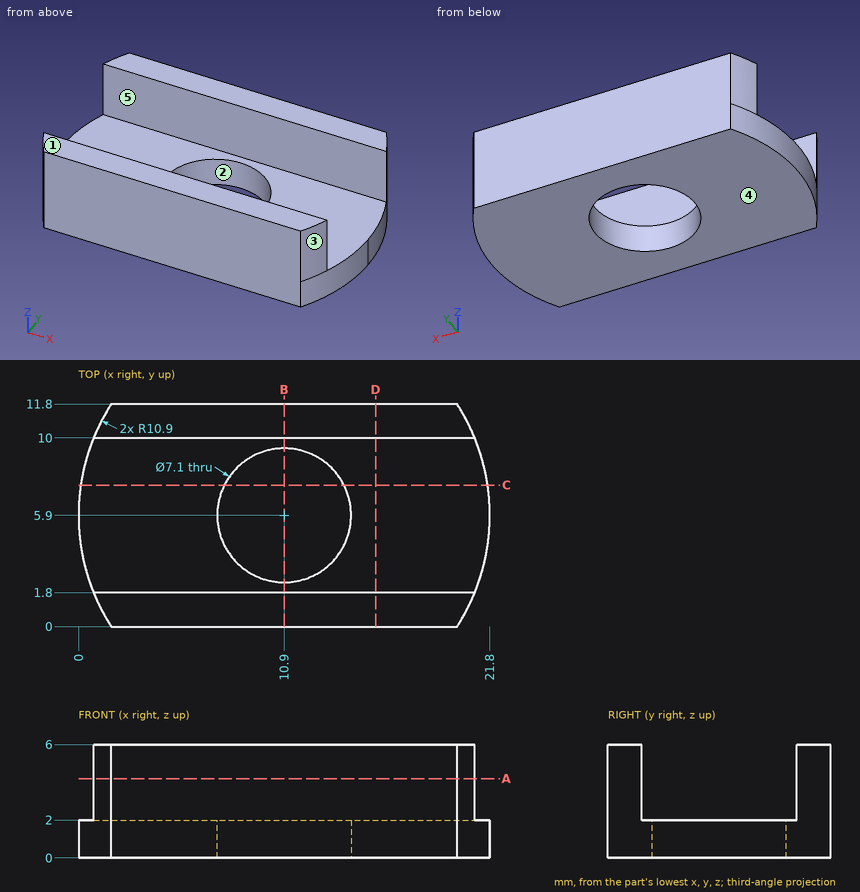
Source: three-view drawing plus pictorial views. Frame: mm from the lowest corner of the part. A direction names the side the tool comes from. Coordinates: 2 decimals unless noted, no trailing zeros. Order: outer loops, then holes, each group sorted by start corner. A loop starts at its lowest first (then second) coordinate and runs counter-clockwise, first axis right, second up. Notation, with made-up numbers: M 54.5,-3.75 L 104.5,-3.75 A15 ccw 104.5,25.25 Z; hole C 56.5,23.5 d9. An arc over 180 degrees is marked long. Write each question's results on one line, items separated by ' | '. Start each with the question number.
1. Section C-C, the plane y = 7.5. Return the cut outline in (x, z).
2. Section A-A, the plane z = 4.2. Return the cut outline in (x, y) (1 decimal), then the cut area to 3 significant figures.
3. Pin query (flat end, axial travel): pin 1 (1 mm diameter, centred on y = 10.5, z = 2, fed in from -X); pin 2 (5 mm diameter, centred on x = 3, y = 7.5, fed in from -Z); pin 3 (1.5 mm diameter, centred on y = 10.5, z = 1, fed in from -X). Return the tip coordinate at first contact, or that it passes through.
4. Reachability of the marked faces 4 and 5 from +Z, -Z, +X, -X, +Y, -Y: full face, straight path, thin tool, end or side. Return the list, or none.
5. Section D-D, the plane x = 15.75. Return the cut outline in (y, z).
6. Section B-B, the plane x = 10.9. Return the cut outline in (y, z), then the cut area to 3 significant figures.
7. Draft query along X for the marked faces 1, 2 and 3. Return one class per face: +X half, -X half, draft (parallel to the pull), parting line (faces both ways), or undercut.
8. Material intervals for L1, parallel to Y at x = 4.75, z = 2.35; L2, parallel to Y at x = 10.9, z = 1.25; L3, parallel to Z at x = 17.25, y = 3.5, sorted ascending.
Solution:
1) outline: M 0.12,0 L 7.73,0 L 7.73,2 L 0.12,2 Z; M 14.07,0 L 21.68,0 L 21.68,2 L 14.07,2 Z
2) outline: M 0.8,1.8 A10.9 ccw 1.7,0 L 20.1,0 A10.9 ccw 21,1.8 Z; M 0.8,10 L 21,10 A10.9 ccw 20.1,11.8 L 1.7,11.8 A10.9 ccw Z | area: 69.6 mm²
3) pin 1: x = 0.8 | pin 2: z = 0 | pin 3: x = 0.7
4) face 4: -Z, +X, -X, +Y, -Y | face 5: +Z, +X, -X
5) outline: M 0,0 L 11.8,0 L 11.8,6 L 10,6 L 10,2 L 1.8,2 L 1.8,6 L 0,6 Z
6) outline: M 0,0 L 2.35,0 L 2.35,2 L 1.8,2 L 1.8,6 L 0,6 Z; M 9.45,0 L 11.8,0 L 11.8,6 L 10,6 L 10,2 L 9.45,2 Z | area: 23.8 mm²
7) face 1: draft | face 2: undercut | face 3: +X half
8) L1: 0 to 1.8, 10 to 11.8 | L2: 0 to 2.35, 9.45 to 11.8 | L3: 0 to 2
